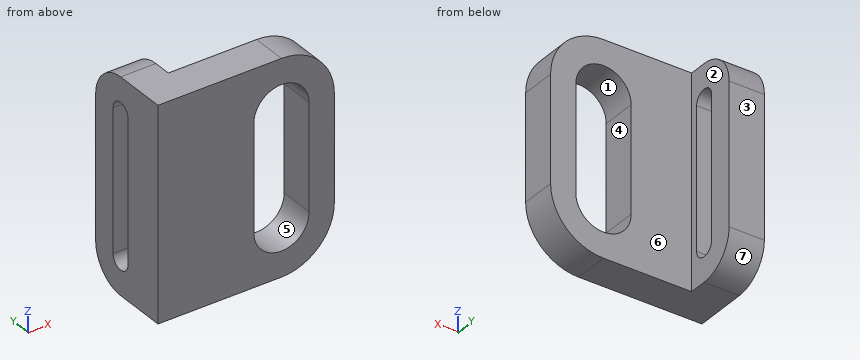
from build123d import *

# Parameters (mm, degrees)
IZIM2_W                     = 80
IZIM2_H                     = 120
IZIM2_W_2                   = 20
Y_KSEKLIK_EKSTR_ZYON3_DEPTH = 20
RADYUS1_R                   = 30
IZIM3_W                     = 20
IZIM3_H                     = 120
EKSTR_ZYON_NCE1_DEPTH       = 50
RADYUS2_R                   = 20
KES_EKSTR_ZYON3_DEPTH       = 20


with BuildPart() as part:
    # Çizim2 → Yükseklik-Ekstrüzyon3 (new body)
    # profile 1 of 2: a face of its own
    with BuildSketch(Plane(origin=(0, 0, 0), x_dir=(1, 0, 0), z_dir=(0, 1, 0))):
        with Locations((-4.018691589, -18.785046729)):
            Rectangle(IZIM2_W, IZIM2_H)
        with BuildLine():
            ThreePointArc((-9.719626168, 11.214953271), (5.981308411, 26.91588785), (21.682242991, 11.214953271))
            Line((21.682242991, 11.214953271), (21.682242991, -48.785046729))
            ThreePointArc((21.682242991, -48.785046729), (5.981308411, -64.485981308), (-9.719626168, -48.785046729))
            Line((-9.719626168, -48.785046729), (-9.719626168, 11.214953271))
        make_face(mode=Mode.SUBTRACT)
    # profile 2 of 2: a face of its own
    with BuildSketch(Plane(origin=(0, 0, 0), x_dir=(1, 0, 0), z_dir=(0, 1, 0))):
        with Locations((-54.018691589, -18.785046729)):
            Rectangle(IZIM2_W_2, IZIM2_H)
    extrude(amount=Y_KSEKLIK_EKSTR_ZYON3_DEPTH)

    # Radyus1
    radyus1_edges = [part.edges().sort_by_distance(p)[0] for p in [
        (35.981308411, 10, -41.214953271),
        (35.981308411, 10, 78.785046729),
    ]]
    fillet(radyus1_edges, radius=RADYUS1_R)

    # Çizim3 → Ekstrüzyon-İnce1 (add)
    with BuildSketch(Plane(origin=(0, 0, 0), x_dir=(1, 0, 0), z_dir=(0, 1, 0))):
        with Locations((-54.018691589, -18.785046729)):
            Rectangle(IZIM3_W, IZIM3_H)
    extrude(amount=EKSTR_ZYON_NCE1_DEPTH)

    # Radyus2
    radyus2_edges = [part.edges().sort_by_distance(p)[0] for p in [
        (-54.018691589, 50, 78.785046729),
        (-54.018691589, 50, -41.214953271),
    ]]
    fillet(radyus2_edges, radius=RADYUS2_R)

    # Çizim6 → Kes-Ekstrüzyon3 (cut)
    with BuildSketch(Plane(origin=(-44.018691589, 0, 0), x_dir=(0, 0, -1), z_dir=(1, 0, 0))):
        with BuildLine():
            Line((-58.785046729, 36), (21.214953271, 36))
            ThreePointArc((21.214953271, 36), (27.214953271, 30), (21.214953271, 24))
            Line((21.214953271, 24), (-58.785046729, 24))
            ThreePointArc((-58.785046729, 24), (-64.785046729, 30), (-58.785046729, 36))
        make_face()
    extrude(amount=-KES_EKSTR_ZYON3_DEPTH, mode=Mode.SUBTRACT)


solid = part.part
CAD build for the part. Positions are in the model's coordinates, mm. Face numbers are marked on the shaded views. A direction names the side the tool comes from. Coordinates: 2 decimals unless noted, no trailing zeros. Write each loop counter-clockwise with the first axis right and the second up, starting at its lowest first coordinate (ties: lowest second). Pieces come first, ordered by that corner, then holes. Notation, with made-up numbers: M 36.25,72.5 L 95.25,72.5 A18 ccw 95.25,82.5 Z; hole C -13.5,-1 d9. An arc over 180 degrees is marked long. Answer as a JSON object with one key per item and string values. Group by question number.
1) Saw through at B-B (x = -55.5). Write the cut outline in (y, z), plus the area to 3 significant figures.
2) Saw through at D-D (x = 10.5). Write the cut outline in (y, z), plus the area to 3 significant figures.
3) Saw through at A-A (z = 3.5). Write the cut outline in (x, y).
4) Wall check: line 1 (X direction, y = 12, z = 20); line 2 (X direction, y = 38, z = 19); line 3 (Y direction, x = -43, z = 8.5). Give the ranges that are in metal, low to high. Write a range as from..to.
5) Pin check, flat tips, straight feed: pin 1 Ø16 at (x, z) = (-58.5, 3.5) entering from -Y; pin 2 Ø5 at (x, y) = (-48.5, 36.5) entering from +Z; pin 3 Ø4 at (y, z) = (35.5, 50.5) entering from +X. Stop position of each tip, or through.
6) Saw through at C-C (y = 10). Write the cut outline in (x, z).
7) Mould opens along X. For the marked faces 1, 2, 3 and 4 say: +X half, -X half, draft (parallel to the pull), parting line (faces both ways), or undercut.
8) Tool access for the marked faces 5, 6 and 7: list every direction of +Z, -Z, +X, -X, +Y, -Y with a clear straight run to the whole face (end or side of a thin tool).
Values follow:
{
 "1": {"outline": "M 0,-41.21 L 30,-41.21 A20 ccw 50,-21.21 L 50,58.79 A20 ccw 30,78.79 L 0,78.79 Z; hole M 24,-21.21 A6 ccw 36,-21.21 L 36,58.79 A6 ccw 24,58.79 Z", "area": "4,760 mm2"},
 "2": {"outline": "M 0,-40.87 L 20,-40.87 L 20,-26.25 L 0,-26.25 Z; M 0,63.82 L 20,63.82 L 20,78.44 L 0,78.44 Z", "area": "585 mm2"},
 "3": {"outline": "M -64.02,0 L -9.72,0 L -9.72,20 L -44.02,20 L -44.02,24 L -64.02,24 Z; M -64.02,36 L -44.02,36 L -44.02,50 L -64.02,50 Z; M 21.68,0 L 35.98,0 L 35.98,20 L 21.68,20 Z"},
 "4": {"line 1": "x = -64.02..-9.72, 21.68..35.98", "line 2": "x = -64.02..-44.02", "line 3": "y = 0..20"},
 "5": {"pin 1": "stops at y = 0", "pin 2": "stops at z = 78.38", "pin 3": "stops at x = -44.02"},
 "6": {"outline": "M -64.02,-41.21 L 5.98,-41.21 A30 ccw 35.98,-11.21 L 35.98,48.79 A30 ccw 5.98,78.79 L -64.02,78.79 Z; hole M -9.72,-11.21 A15.7 ccw 21.68,-11.21 L 21.68,48.79 A15.7 ccw -9.72,48.79 Z"},
 "7": {"face 1": "undercut", "face 2": "+X half", "face 3": "draft", "face 4": "undercut"},
 "8": {"face 5": "+Y, -Y", "face 6": "+Z, -Z, +X, +Y", "face 7": "-Z, +X, -X, +Y"}
}
